```python
from build123d import *

# Parameters (mm, degrees)
SKETCH1_W                  = 40
SKETCH1_H                  = 106
BOSS_EXTRUDE1_DEPTH        = 8.5
SKETCH2_W                  = 35
SKETCH2_H                  = 70
CUT_EXTRUDE1_DEPTH         = 3
SKETCH3_W                  = 10.5
SKETCH3_H                  = 10
CUT_EXTRUDE2_DEPTH         = 1.35
SKETCH4_W                  = 12.5
SKETCH4_H                  = 6
CUT_EXTRUDE3_DEPTH         = 3.1
SKETCH5_W                  = 8.5
SKETCH5_H                  = 17.5
PCB_PLACE_DEPTH            = 3.1
SKETCH6_W                  = 8.5
SKETCH6_H                  = 1.6
NICKEL_STRIP_HOLE_DEPTH    = 70.174850921
CUT_EXTRUDE4_REACH         = 71.486
SKETCH7_W                  = 8.5
SKETCH7_H                  = 17.5
SKETCH8_W                  = 8.5
SKETCH8_H                  = 1.6
CUT_EXTRUDE5_DEPTH         = 10
SKETCH9_W                  = 8.5
SKETCH9_H                  = 106
NICKEL_STRIP_RAIL_DEPTH    = 2.5
FILLET3_R                  = 2.325
FILLET4_RADIUS             = 1.45
FILLET4_LENGTH             = 8.5
SKETCH10_W                 = 8.5
SKETCH10_H                 = 5
CUT_EXTRUDE6_DEPTH         = 1.5
SKETCH11_W                 = 8.5
SKETCH11_H                 = 0.7
NICKELSTRIPINSERTION_DEPTH = 18
FILLET5_INSERTION_START    = -10.9
FILLET5_INSERTION_DEPTH    = 8.5
FILLET5_INSERTION_START_2  = 2.4
FILLET5_INSERTION_2_DEPTH  = 8.5
FILLET7_AMEND_R            = 4
FILLET6_START              = -10.9
FILLET6_DEPTH              = 8.5
FILLET6_START_2            = 2.4
FILLET6_2_DEPTH            = 8.5
FILLET8_ROUNDING_R         = 0.1
SKETCH12_W                 = 0.3
SKETCH12_H                 = 0.8
STRIPRAIL_DEPTH            = 70
SKETCH13_R                 = 1.75
SCREW_HOLES_DEPTH          = 70.485610128
SKETCH14_R                 = 3.5
SCREW_HEAD_HOLES_TBM_DEPTH = 3.5


with BuildPart() as part:
    # Sketch1 → Boss-Extrude1 (new body)
    with BuildSketch(Plane(origin=(0, 0, 0), x_dir=(1, 0, 0), z_dir=(0, 1, 0))):
        with Locations((0, 13)):
            Rectangle(SKETCH1_W, SKETCH1_H)
    extrude(amount=BOSS_EXTRUDE1_DEPTH)

    # Sketch2 → Cut-Extrude1 (cut)
    with BuildSketch(Plane(origin=(0, 8.5, 0), x_dir=(1, 0, 0), z_dir=(0, 1, 0))):
        with Locations((0, 2)):
            Rectangle(SKETCH2_W, SKETCH2_H)
    extrude(amount=-CUT_EXTRUDE1_DEPTH, mode=Mode.SUBTRACT)

    # Sketch3 → Cut-Extrude2 (cut)
    with BuildSketch(Plane(origin=(0, 8.5, 0), x_dir=(1, 0, 0), z_dir=(0, 1, 0))):
        with Locations((-6.65, 42)):
            Rectangle(SKETCH3_W, SKETCH3_H)
        with Locations((6.65, 42)):
            Rectangle(SKETCH3_W, SKETCH3_H)
    extrude(amount=-CUT_EXTRUDE2_DEPTH, mode=Mode.SUBTRACT)

    # Sketch4 → Cut-Extrude3 (cut)
    with BuildSketch(Plane(origin=(0, 8.5, 0), x_dir=(1, 0, 0), z_dir=(0, 1, 0))):
        with Locations((6.65, 44)):
            Rectangle(SKETCH4_W, SKETCH4_H)
    extrude(amount=-CUT_EXTRUDE3_DEPTH, mode=Mode.SUBTRACT)

    # Sketch5 → PCB place (cut)
    with BuildSketch(Plane(origin=(0, 8.5, 0), x_dir=(1, 0, 0), z_dir=(0, 1, 0))):
        with Locations((6.65, 55.75)):
            Rectangle(SKETCH5_W, SKETCH5_H)
    extrude(amount=-PCB_PLACE_DEPTH, mode=Mode.SUBTRACT)

    # Sketch6 → Nickel strip hole (cut, through all)
    with BuildSketch(Plane(origin=(0, 5.4, 0), x_dir=(1, 0, 0), z_dir=(0, 1, 0))):
        with Locations((6.65, 63.7)):
            Rectangle(SKETCH6_W, SKETCH6_H)
    extrude(amount=-NICKEL_STRIP_HOLE_DEPTH, mode=Mode.SUBTRACT)

    # Cut-Extrude4: up to this face of the body (flat: up to its plane)
    cut_extrude4_end = Plane(part.part.faces().sort_by_distance((6.65, 5.4, -51.042077088))[0])
    # Sketch7 → Cut-Extrude4 (cut, up to the picked face)
    with BuildSketch(Plane(origin=(0, 8.5, 0), x_dir=(1, 0, 0), z_dir=(0, 1, 0)), mode=Mode.PRIVATE) as cut_extrude4_sk1:
        with Locations((-6.65, 55.75)):
            Rectangle(SKETCH7_W, SKETCH7_H)
    cut_extrude4_tool1 = split(extrude(cut_extrude4_sk1.sketch, amount=-CUT_EXTRUDE4_REACH, mode=Mode.PRIVATE), bisect_by=cut_extrude4_end, keep=Keep.BOTH, mode=Mode.PRIVATE)
    add(cut_extrude4_tool1.solids().sort_by(Axis((-6.65, 8.5, -55.75), (0, -1, 0)))[0], mode=Mode.SUBTRACT)

    # Sketch8 → Cut-Extrude5 (cut)
    with BuildSketch(Plane(origin=(0, 5.4, 0), x_dir=(1, 0, 0), z_dir=(0, 1, 0))):
        with Locations((-6.65, 47.8)):
            Rectangle(SKETCH8_W, SKETCH8_H)
    extrude(amount=-CUT_EXTRUDE5_DEPTH, mode=Mode.SUBTRACT)

    # Sketch9 → Nickel strip rail (cut)
    with BuildSketch(Plane.XZ):
        with Locations((-6.65, -13)):
            Rectangle(SKETCH9_W, SKETCH9_H)
        with Locations((6.65, -13)):
            Rectangle(SKETCH9_W, SKETCH9_H)
    extrude(amount=-NICKEL_STRIP_RAIL_DEPTH, mode=Mode.SUBTRACT)

    # Fillet3
    # the kernel refuses this fillet: 2.325 mm, written as the material it takes off along each edge
    with BuildSketch(Plane(origin=(3.4125, 7.15, -47), x_dir=(0, 0, 1), z_dir=(-1, 0, 0))) as fillet3_piece_1_section:
        with BuildLine():
            CenterArc((FILLET3_R, -FILLET3_R), FILLET3_R, 90, 90)
            Line((0, -FILLET3_R), (0, 0))
            Line((0, 0), (FILLET3_R, 0))
        make_face()
    fillet3_piece_1 = extrude(amount=20.125, mode=Mode.PRIVATE)
    fillet3_piece_1 = split(fillet3_piece_1, bisect_by=Plane(origin=(-11.9, 7.15, -47), z_dir=(1, 0, 0)), keep=Keep.TOP, mode=Mode.PRIVATE)
    fillet3_piece_1 = split(fillet3_piece_1, bisect_by=Plane(origin=(-1.4, 7.15, -47), z_dir=(-1, 0, 0)), keep=Keep.TOP, mode=Mode.PRIVATE)
    add(fillet3_piece_1, mode=Mode.SUBTRACT)
    with BuildSketch(Plane(origin=(-10.9, 2.5, -47), x_dir=(0, 1, 0), z_dir=(1, 0, 0))) as fillet3_piece_2:
        with BuildLine():
            CenterArc((FILLET3_R, FILLET3_R), FILLET3_R, 180, 90)
            Line((0, FILLET3_R), (0, 0))
            Line((0, 0), (FILLET3_R, 0))
        make_face()
    extrude(amount=8.5, mode=Mode.SUBTRACT)

    # Fillet4: full round fillet: the end face becomes a half cylinder, R = half its width
    fillet4_face = Plane((6.65, 3.95, -62.9), x_dir=(1, 0, 0), z_dir=(0, 0, -1))  # on the end face: x along it, z out of the body
    fillet4_slab = fillet4_face.offset(-FILLET4_RADIUS / 2) * Box(FILLET4_LENGTH, 2 * FILLET4_RADIUS, FILLET4_RADIUS, mode=Mode.PRIVATE)  # the body's end, R deep
    fillet4_round = Plane((6.65, 3.95, -61.45), x_dir=(0, 0, -1), z_dir=(1, 0, 0)) * Cylinder(FILLET4_RADIUS, FILLET4_LENGTH, mode=Mode.PRIVATE)  # its axis R under the face
    add(fillet4_slab - fillet4_round, mode=Mode.SUBTRACT)

    # Sketch10 → Cut-Extrude6 (cut)
    with BuildSketch(Plane.XZ.offset(-2.5)):
        with Locations((6.65, 6.5)):
            Rectangle(SKETCH10_W, SKETCH10_H)
        with Locations((-6.65, 6.5)):
            Rectangle(SKETCH10_W, SKETCH10_H)
    extrude(amount=-CUT_EXTRUDE6_DEPTH, mode=Mode.SUBTRACT)

    # Sketch11 → NickelStripInsertion (cut)
    with BuildSketch(Plane(origin=(0, 0, 9), x_dir=(-1, 0, 0), z_dir=(0, 0, -1))):
        with Locations((-6.65, 3.65)):
            Rectangle(SKETCH11_W, SKETCH11_H)
        with Locations((6.65, 3.65)):
            Rectangle(SKETCH11_W, SKETCH11_H)
    extrude(amount=-NICKELSTRIPINSERTION_DEPTH, mode=Mode.SUBTRACT)

    # Fillet5_insertion: read off the stored shape, not the designer's step
    # Fillet5_insertion outline → Fillet5_insertion (cut)
    with BuildSketch(Plane.YZ.offset(FILLET5_INSERTION_START)):
        with BuildLine():
            Line((2.5, 4), (2.5, -8.359207094))
            add(Edge.make_bspline(
                [(2.5, -8.359207094), (2.5, 2.968380423), (4, 4)],
                knots=[0, 0, 0, 1, 1, 1], degree=2, weights=[1, 0.885061203, 1]))
            Line((4, 4), (2.5, 4))
        make_face()
    extrude(amount=FILLET5_INSERTION_DEPTH, mode=Mode.SUBTRACT)

    # Fillet5_insertion 2 outline → Fillet5_insertion 2 (cut)
    with BuildSketch(Plane.YZ.offset(FILLET5_INSERTION_START_2)):
        with BuildLine():
            Line((2.5, 4), (2.5, -8.359207094))
            add(Edge.make_bspline(
                [(2.5, -8.359207094), (2.5, 2.968380423), (4, 4)],
                knots=[0, 0, 0, 1, 1, 1], degree=2, weights=[1, 0.885061203, 1]))
            Line((4, 4), (2.5, 4))
        make_face()
    extrude(amount=FILLET5_INSERTION_2_DEPTH, mode=Mode.SUBTRACT)

    # Fillet7_amend
    fillet7_amend_edges = [part.edges().sort_by_distance(p)[0] for p in [
        (6.65, 4, 4),
        (-6.65, 4, 4),
    ]]
    fillet(fillet7_amend_edges, radius=FILLET7_AMEND_R)

    # Fillet6: read off the stored shape, not the designer's step
    # Fillet6 outline → Fillet6 (cut)
    with BuildSketch(Plane.YZ.offset(FILLET6_START)):
        with BuildLine():
            Line((3.3, 9), (3.3, 16.909487973))
            add(Edge.make_bspline(
                [(3.3, 16.909487973), (3.3, 9.121373217), (2.5, 9)],
                knots=[0, 0, 0, 1, 1, 1], degree=2, weights=[1, 0.758287544, 1]))
            Line((2.5, 9), (3.3, 9))
        make_face()
    extrude(amount=FILLET6_DEPTH, mode=Mode.SUBTRACT)

    # Fillet6 2 outline → Fillet6 2 (cut)
    with BuildSketch(Plane.YZ.offset(FILLET6_START_2)):
        with BuildLine():
            Line((3.3, 9), (3.3, 16.909487973))
            add(Edge.make_bspline(
                [(3.3, 16.909487973), (3.3, 9.121373217), (2.5, 9)],
                knots=[0, 0, 0, 1, 1, 1], degree=2, weights=[1, 0.758287544, 1]))
            Line((2.5, 9), (3.3, 9))
        make_face()
    extrude(amount=FILLET6_2_DEPTH, mode=Mode.SUBTRACT)

    # Fillet8_rounding
    fillet8_rounding_edges = [part.edges().sort_by_distance(p)[0] for p in [
        (-6.65, 2.5, 9),
        (6.65, 2.5, 9),
    ]]
    fillet(fillet8_rounding_edges, radius=FILLET8_ROUNDING_R)

    # Sketch12 → StripRail (add)
    with BuildSketch(Plane.XY.offset(40)):
        with Locations((2.55, 0.4)):
            Rectangle(SKETCH12_W, SKETCH12_H)
        with Locations((-10.75, 0.4)):
            Rectangle(SKETCH12_W, SKETCH12_H)
        with Locations((-2.55, 0.4)):
            Rectangle(SKETCH12_W, SKETCH12_H)
        with Locations((10.75, 0.4)):
            Rectangle(SKETCH12_W, SKETCH12_H)
    extrude(amount=-STRIPRAIL_DEPTH)

    # Sketch13 → Screw_Holes (cut, through all)
    with BuildSketch(Plane.XZ):
        with Locations(Location((-16, -61, 0), (0, 0, 270))):
            Circle(SKETCH13_R)
        with Locations(Location((16, -61, 0), (0, 0, 270))):
            Circle(SKETCH13_R)
        with Locations(Location((-16, 36, 0), (0, 0, 270))):
            Circle(SKETCH13_R)
        with Locations(Location((16, 36, 0), (0, 0, 270))):
            Circle(SKETCH13_R)
    extrude(amount=-SCREW_HOLES_DEPTH, mode=Mode.SUBTRACT)

    # Sketch14 → Screw_Head_Holes_TBM (cut)
    with BuildSketch(Plane.XZ):
        with Locations(Location((16, -61, 0), (0, 0, 270))):
            Circle(SKETCH14_R)
        with Locations(Location((-16, -61, 0), (0, 0, 270))):
            Circle(SKETCH14_R)
        with Locations(Location((16, 36, 0), (0, 0, 270))):
            Circle(SKETCH14_R)
        with Locations(Location((-16, 36, 0), (0, 0, 270))):
            Circle(SKETCH14_R)
    extrude(amount=-SCREW_HEAD_HOLES_TBM_DEPTH, mode=Mode.SUBTRACT)


solid = part.part
```
Verification items for the finished model (mm, model axes). A direction names the side the tool comes from. Coordinates: 2 decimals unless noted, no trailing zeros. Order: outer loops, then holes, each group sorted by start corner. A loop starts at its lowest first (then second) coordinate and runs counter-clockwise, first axis right, second up. Notation, with made-up numbers: (70, 21) -> (115, 21) arc R14 ccw to (115, 42) -> close; hole circle Ø8 at (26.5, 84.5). An arc over 180 degrees is marked (long way). Put each result on its own line as item: value. Start each with the question number.
1) Go/stop test with a flat-tipped pin: pin 1 (7 mm diameter, centred on x = 7.5, z = 22.5, fed in from +Y). Record where the tip stops, or that it passes through.
2) Release check for a two-part mould opening along X. For faces 6 (the flat face through (-15, 0, -14)), 7 (the cylindrical face through (-15.474, 5.965, -62.669)) record: pulls with the +X half, pulls with the -X half, needs draft (parallel to the pull), parting line crosses it, or undercut.
3) Tool access check on faces 1 (the flat face through (7, 4, 16)), 2 (the flat face through (0, 5, 40)), 3 (the flat face through (7, 7.15, -39)), 4 (the flat face through (0, 5, -66)), 5 (the cylindrical face through (-15.846, 1.726, 39.497)). Record the directions out of +Z, -Z, +X, -X, +Y, -Y that give a thin tool (end or side, any length) a straight path to the whole face; none if there is none.
4) Material ranges on L1, parallel to X at y = 2, z = -45; L2, parallel to X at y = 6.5, z = -61; L3, parallel to X at y = 0.75, z = 14.5, recorded low to high.
5) Cross-section at A-A (x = 16). Enter the section's corners in (y, z).
6) Cross-section at B-B (z = -23.5). Enter the section's corners in (x, y), plus the area to 3 significant figures.
Geometry check:
1. pin 1: stops at y = 5.5
2. face 6: needs draft
2. face 7: undercut
3. face 1: none
3. face 2: +Z, +X, -X, +Y, -Y
3. face 3: +Y
3. face 4: -Z, +X, -X, +Y, -Y
3. face 5: -Y
4. L1: x = -20 to -10.9, -2.4 to 2.4, 10.9 to 20
4. L2: x = -20 to -17.75, -14.25 to -10.9, -2.4 to 2.4, 10.9 to 14.25, 17.75 to 20
4. L3: x = -20 to -10.6, -2.7 to 2.7, 10.6 to 20
5. outline: (0, -66) -> (8.5, -66) -> (8.5, -62.75) -> (3.5, -62.75) -> (3.5, -64.5) -> (0, -64.5) -> close; (0, -57.5) -> (3.5, -57.5) -> (3.5, -59.25) -> (8.5, -59.25) -> (8.5, -37) -> (5.5, -37) -> (5.5, 33) -> (8.5, 33) -> (8.5, 34.25) -> (3.5, 34.25) -> (3.5, 32.5) -> (0, 32.5) -> close; (0, 39.5) -> (3.5, 39.5) -> (3.5, 37.75) -> (8.5, 37.75) -> (8.5, 40) -> (0, 40) -> close
6. outline: (-20, 0) -> (-10.6, 0) -> (-10.6, 0.8) -> (-10.9, 0.8) -> (-10.9, 2.5) -> (-2.4, 2.5) -> (-2.4, 0.8) -> (-2.7, 0.8) -> (-2.7, 0) -> (2.7, 0) -> (2.7, 0.8) -> (2.4, 0.8) -> (2.4, 2.5) -> (10.9, 2.5) -> (10.9, 0.8) -> (10.6, 0.8) -> (10.6, 0) -> (20, 0) -> (20, 8.5) -> (17.5, 8.5) -> (17.5, 5.5) -> (-17.5, 5.5) -> (-17.5, 8.5) -> (-20, 8.5) -> close
6. area: 193 mm^2
